```python
from build123d import *

# Parameters (mm, degrees)
SKETCH2_R                         = 12.7
BOSS_EXTRUDE1_DEPTH               = 9.525
PIPE_TAP_DRILL_FOR_1_2_TAP1_D     = 17.8562
PIPE_TAP_DRILL_FOR_1_2_TAP1_DEPTH = 31.75
PIPE_TAP_DRILL_FOR_1_2_TAP1_TIP   = 5.364543693


with BuildPart() as part:
    # Sketch1 → Revolve1 (revolve)
    with BuildSketch(Plane.XY):
        Polygon((-101.6, 0), (-101.6, -12.7), (-48.821281066, -12.7), (-48.821281066, -10.922), (-46.281281066, -10.922), (-46.281281066, -12.7), (-44.45, -12.7), (-44.45, -6.35), (0, -6.35), (0, 0), align=None)
    revolve(axis=Axis((0, -6.35, 0), (0, 1, 0)))

    # Sketch2 → Boss-Extrude1 (add)
    with BuildSketch(Plane(origin=(0, 0, 0), x_dir=(1, 0, 0), z_dir=(0, 1, 0))):
        Circle(SKETCH2_R)
    extrude(amount=BOSS_EXTRUDE1_DEPTH)

    # Pipe Tap Drill for 1/2 Tap1
    with Locations(Plane(origin=(0, 9.525, 0), x_dir=(1, 0, 0), z_dir=(0, 1, 0))):
        with Locations((0, 0)):
            Hole(PIPE_TAP_DRILL_FOR_1_2_TAP1_D / 2, depth=PIPE_TAP_DRILL_FOR_1_2_TAP1_DEPTH)
            with Locations((0, 0, -(PIPE_TAP_DRILL_FOR_1_2_TAP1_DEPTH + PIPE_TAP_DRILL_FOR_1_2_TAP1_TIP / 2))):  # 118° drill point
                Cone(0, PIPE_TAP_DRILL_FOR_1_2_TAP1_D / 2, PIPE_TAP_DRILL_FOR_1_2_TAP1_TIP, mode=Mode.SUBTRACT)


solid = part.part
```
The model under review builds one solid part; all positions refer to its coordinate system, in mm. A direction names the side the tool comes from. Round coordinates to 2 decimals unless told otherwise and drop trailing zeros. Write each loop counter-clockwise with the first axis right and the second up, starting at its lowest first coordinate (ties: lowest second). Pieces come first, ordered by that corner, then holes.
(1) Insertion check: pin 1 (8 mm diameter, centred on x = -61.5, z = -15.5, fed in from +Y); pin 2 (6 mm diameter, centred on x = 68, y = 2, fed in from +Z); pin 3 (2 mm diameter, centred on y = -3.5, z = -74.5, fed in from +X); pin 4 (20.5 mm diameter, centred on x = 0, z = 0, fed in from +Y) (3 decimals). Each pin has a flat end and moves straight along its axis. Give the tip position at first contact, or say it passes through.
(2) We need section C-C on y = -4. Give the boundary of the cut face in (x, z).
(3) We need section A-A on x = 0. Give the boundary of the cut face in (y, z) (3 decimals), and give its area (3 significant figures).
(4) Wall thickness on L1, parallel to Z at x = 0, y = -12.2; L2, parallel to Z at x = 0, y = -7.25; L3, parallel to Z at x = 0.5, y = 7.25: over which ranges is each line inside the solid? List them lowest first.
(5) Mouldability with a two-part tool opening along Z and no side actions: class faces 3 (the cylindrical face through (-2.75, 4.7, 12.4)), 4 (the flat face through (21, 0, 1)), 5 (the flat face through (-18, -10.922, -43)) as +Z half, -Z half, draft (parallel to the pull), parting line (faces both ways), or undercut.
(6) Machinability: for faces 1 (the flat face through (17.4, -12.7, 41.4)), 2 (the cylindrical face through (-44.144, -11.823, 13.902)), which of the approach directions +Z, -Z, +X, -X, +Y, -Y give a long, thin tool a straight path to every point of the face, cutting with its end or side? Answer none if there is none.
(7) We need section B-B on z = 0. Give the boundary of the cut face in (x, y) (3 decimals).
(8) We need section D-D on x = 22. Give the boundary of the cut face in (y, z), and give its area (3 significant figures).
Findings below:
1. pin 1: stops at y = 0
1. pin 2: stops at z = 77.44
1. pin 3: stops at x = 70.14
1. pin 4: stops at y = 9.525
2. outline: circle Ø203.2 at (0, 0); hole circle Ø17.86 at (0, 0)
3. outline: (-12.7, -101.6) - (0, -101.6) - (0, -12.7) - (9.525, -12.7) - (9.525, -8.928) - (-6.35, -8.928) - (-6.35, -44.45) - (-12.7, -44.45) - (-12.7, -46.281) - (-10.922, -46.281) - (-10.922, -48.821) - (-12.7, -48.821) - close; (-12.7, 44.45) - (-6.35, 44.45) - (-6.35, 8.928) - (9.525, 8.928) - (9.525, 12.7) - (0, 12.7) - (0, 101.6) - (-12.7, 101.6) - (-12.7, 48.821) - (-10.922, 48.821) - (-10.922, 46.281) - (-12.7, 46.281) - close
3. area: 1,970 mm2
4. L1: z = -101.6 to -48.82, -46.28 to -44.45, 44.45 to 46.28, 48.82 to 101.6
4. L2: z = -101.6 to -44.45, 44.45 to 101.6
4. L3: z = -12.69 to -8.91, 8.91 to 12.69
5. face 3: parting line
5. face 4: draft
5. face 5: undercut
6. face 1: +Z, -Z, +X, -X, -Y
6. face 2: -Y
7. outline: (-101.6, -12.7) - (-48.821, -12.7) - (-48.821, -10.922) - (-46.281, -10.922) - (-46.281, -12.7) - (-44.45, -12.7) - (-44.45, -6.35) - (-8.928, -6.35) - (-8.928, 9.525) - (-12.7, 9.525) - (-12.7, 0) - (-101.6, 0) - close; (8.928, -6.35) - (44.45, -6.35) - (44.45, -12.7) - (46.281, -12.7) - (46.281, -10.922) - (48.821, -10.922) - (48.821, -12.7) - (101.6, -12.7) - (101.6, 0) - (12.7, 0) - (12.7, 9.525) - (8.928, 9.525) - close
8. outline: (-12.7, -99.19) - (0, -99.19) - (0, 99.19) - (-12.7, 99.19) - (-12.7, 43.58) - (-10.92, 43.58) - (-10.92, 40.72) - (-12.7, 40.72) - (-12.7, 38.62) - (-6.35, 38.62) - (-6.35, -38.62) - (-12.7, -38.62) - (-12.7, -40.72) - (-10.92, -40.72) - (-10.92, -43.58) - (-12.7, -43.58) - close
8. area: 2,020 mm2
